```python
from build123d import *

# Parameters (mm, degrees)
F1_DEPTH = 25.4
F2_R     = 5.08
F3_T     = -2.54


# Not quite as in the source:
# - a shell that OpenCascade refuses in one call is made with other operations: the cavity is built on its own and cut out


with BuildPart() as f1:
    # F0 (on Front) → F1 (new body)
    with BuildSketch(Plane.XZ):
        Polygon((35.6235019863, 0), (-18.2880014181, 47.0535010099), (-24.5744995773, 0), align=None)
    extrude(amount=F1_DEPTH)

    # F2
    f2_edges = [f1.edges().sort_by_distance(p)[0] for p in [
        (8.66775, -25.4, 23.526751),
        (-21.43125, -25.4, 23.526751),
        (5.524501, -25.4, 0),
        (35.623502, -12.7, 0),
        (8.66775, 0, 23.526751),
        (-21.43125, 0, 23.526751),
        (5.524501, 0, 0),
    ]]
    fillet(f2_edges, radius=F2_R)

    # F3: a shell. OpenCascade refuses it in one call, so the cavity is built on its own and cut out:
    # the body offset inwards by the wall thickness, plus a prism from it out through each open face.
    f3_core = offset(f1.part, amount=F3_T, mode=Mode.PRIVATE)
    f3_exits = [f3_core.faces().sort_by_distance(p)[0] for p in [
        (-3.732644, -2.54, 15.722949),
        (-3.732644, -22.86, 15.722949),
    ]]
    add(f3_core, mode=Mode.SUBTRACT)
    extrude(f3_exits, amount=-F3_T, mode=Mode.SUBTRACT)


solid = f1.part
```
The model under review builds one solid part; all positions refer to its coordinate system, in mm. A direction names the side the tool comes from. Give positions to 0.01 mm unless a question says otherwise; leave off trailing zeros. Write each loop counter-clockwise with the first axis right and the second up, starting at its lowest first coordinate (ties: lowest second). Pieces come first, ordered by that corner, then holes. Notation, with made-up numbers: (-29, -29.5) - (-9, -29.5) arc R9 ccw to (-9, -18.5) - close; hole circle Ø6 at (66.5, 29). An arc over 180 degrees is marked (long way). Answer in a Markdown table with one row per item. Add a question column.
1. Insertion check: P1, Ø5, axis at x = -10, y = -22, coming from the +Z side; P2, Ø6, axis at x = -14, y = -22, coming from the +Z side; P3, Ø8, axis at x = -5, z = 34.5, coming from the -Y side. Each pin has a flat end and moves straight along its axis. Give the tip position at first contact, or say it passes through.
2. We need section B-B on y = -21.5. Write out the cut boundary in (x, z).
3. We need section A-A on y = -9. Write out the cut boundary in (x, z).
4. Wall thickness on line 1 along X through (y, z) = (-14.25, 23.5); line 2 along X through (y, z) = (-23, 8); line 3 along Z through (x, y) = (24, -6.5): over which ranges is each line inside the solid? List them lowest first. Write a range as [from, to].
5. Tool access review of faces 1 (the cylindrical face through (2.918, -22.096, 24.212)), 2 (the cylindrical face through (-20.04, -1.53, 23.01)), 3 (the flat face through (-16.608, -24.112, 21.268)): name each direction out of +Z, -Z, +X, -X, +Y, -Y from which nothing blocks a thin tool from reaching the whole face with its end or side.
6. Draft analysis for pull direction Z (two halves, no side actions). For faces 4 (the flat face through (-2, -13, 0)), 5 (the cylindrical face through (-18.35, -22.1, 21.91)), 6 (the flat face through (-21.387, -12.593, 23.856)), state which applies: +Z half, -Z half, draft (parallel to the pull), parting line (faces both ways), or undercut.
Ans:
| question | item | result |
|---|---|---|
| 1 | P1 | stops at z = 41.79 |
| 1 | P2 | stops at z = 45.73 |
| 1 | P3 | stops at y = -25.39 |
| 2 | outline | (-24.42, 0.14) - (22.08, 0.14) arc R4.94 ccw to (25.33, 8.8) - (-18.18, 46.78) - close; hole (-21.34, 2.83) - (22.08, 2.83) arc R2.25 ccw to (23.56, 6.77) - (-16.18, 41.46) - close |
| 3 | outline | (-24.57, 0) - (22.08, 0) arc R5.08 ccw to (25.42, 8.91) - (-18.29, 47.05) - close; hole (-21.67, 2.54) - (22.08, 2.54) arc R2.54 ccw to (23.75, 6.99) - (-16.4, 42.03) - close |
| 4 | line 1 | x = [-21.43, -18.87], [4.84, 8.7] |
| 4 | line 2 | x = [-22.73, -18.38], [18.73, 25.26] |
| 4 | line 3 | z = [0.38, 3.42], [6.74, 10.14] |
| 5 | face 1 | none |
| 5 | face 2 | +Z, -X, +Y |
| 5 | face 3 | +Y, -Y |
| 6 | face 4 | -Z half |
| 6 | face 5 | undercut |
| 6 | face 6 | +Z half |
